Build history of the part. All positions in model axes, mm. A direction names the side the tool comes from. Coordinates: 2 decimals unless noted, no trailing zeros. Order: outer loops, then holes, each group sorted by start corner. A loop starts at its lowest first (then second) coordinate and runs counter-clockwise, first axis right, second up. Notation, with made-up numbers: (64.25, -22.75) -> (123.25, -22.75) arc R16 cw to (123.25, -10.75) -> close; hole circle Ø2 at (-24.5, 14). An arc over 180 degrees is marked (long way). Write each question's results on one line, items separated by ' | '.
from build123d import *
from build123d.topology import SkipClean

# Parameters (mm, degrees)
SKETCH1_W           = 12
SKETCH1_H           = 9
CUT_EXTRUDE1_START  = 1.272656
CUT_EXTRUDE1_DEPTH  = 0.424218618
CUT_EXTRUDE2_DEPTH  = 5.575781382
SKETCH4_R           = 6.3565957
BOSS_EXTRUDE1_DEPTH = 1.811506156
BOSS_EXTRUDE1_TAPER = 11.136309431
SKETCH5_R           = 6
BOSS_EXTRUDE2_DEPTH = 138.188493844
CHAMFER1_SIZE       = 1.0735
FILLET1_R           = 0.6
FILLET2_R           = 1.2


with BuildPart() as part:
    # Sketch1 → Revolve1 (revolve)
    with BuildSketch(Plane.XY, mode=Mode.PRIVATE) as revolve1_sk:
        with Locations((-6, 4.5)):
            Rectangle(SKETCH1_W, SKETCH1_H)
    revolve(revolve1_sk.sketch.rotate(Axis((-12, 0, 0), (1, 0, 0)), 270), axis=Axis((-12, 0, 0), (1, 0, 0)))

    # Sketch2 → Cut-Extrude1 (cut)
    with BuildSketch(Plane.ZY.offset(10.727344145).offset(CUT_EXTRUDE1_START)):
        Polygon((-2.541695199, 4.306054284), (-2.494007969, 4.33358652), (-2.458304232, 4.354200082), (0, 5.773502692), (2.458305244, 4.354200082), (2.505992237, 4.326667984), (2.541695697, 4.306054284), (5, 2.886751346), (5, 0.048145191), (5, -0.00115583), (5, -0.048145419), (5, -2.886751346), (2.541695697, -4.306053956), (2.494008981, -4.333586191), (2.458305244, -4.354199753), (0, -5.773502692), (-2.458304232, -4.354199753), (-2.505991462, -4.326667518), (-2.541695199, -4.306053956), (-5, -2.886751346), (-5, -0.048145419), (-5, -0.00115583), (-5, 0.048145191), (-5, 2.886751346), align=None)
    extrude(amount=-CUT_EXTRUDE1_DEPTH, mode=Mode.SUBTRACT)

    # Sketch3 → Cut-Extrude2 (cut)
    with SkipClean():  # the faces are left unmerged after this step: merging them gives an invalid solid
        with BuildSketch(Plane.ZY.offset(11.575781382)):
            Polygon((0, 5.773502692), (-5, 2.886751346), (-5, -2.886751346), (0, -5.773502692), (5, -2.886751346), (5, 2.886751346), align=None)
        extrude(amount=-CUT_EXTRUDE2_DEPTH, mode=Mode.SUBTRACT)

    # Sketch4 → Boss-Extrude1 (add)
    with SkipClean():  # the faces are left unmerged after this step: merging them gives an invalid solid
        with BuildSketch(Plane(origin=(0, 0, 0), x_dir=(0, 0, -1), z_dir=(1, 0, 0))):
            Circle(SKETCH4_R)
        extrude(amount=BOSS_EXTRUDE1_DEPTH, taper=BOSS_EXTRUDE1_TAPER)

    # Sketch5 → Boss-Extrude2 (add)
    with SkipClean():  # the faces are left unmerged after this step: merging them gives an invalid solid
        with BuildSketch(Plane(origin=(1.811506156, 0, 0), x_dir=(0, 0, -1), z_dir=(1, 0, 0))):
            Circle(SKETCH5_R)
        extrude(amount=BOSS_EXTRUDE2_DEPTH)

    # Sketch6 → Cut-Revolve1 (revolve, cut)
    with SkipClean():  # the faces are left unmerged after this step: merging them gives an invalid solid
        with BuildSketch(Plane.XY, mode=Mode.PRIVATE) as cut_revolve1_sk:
            Polygon((-6, 5), (-6, 0), (-3.113248654, 0), align=None)
        revolve(cut_revolve1_sk.sketch.rotate(Axis((-6, 0, 0), (1, 0, 0)), 90), axis=Axis((-6, 0, 0), (1, 0, 0)), mode=Mode.SUBTRACT)

    # Chamfer1
    chamfer1_edges = [part.edges().sort_by_distance(p)[0] for p in [
        (140, 0, 6),
    ]]
    chamfer(chamfer1_edges, length=CHAMFER1_SIZE)

    # Fillet1
    fillet1_edges = [part.edges().sort_by_distance(p)[0] for p in [
        (0, 0, 6.3565957),
        (1.811506156, 0, 6),
    ]]
    fillet(fillet1_edges, radius=FILLET1_R)

    # Fillet2
    fillet2_edges = [part.edges().sort_by_distance(p)[0] for p in [
        (-12, 0, 9),
    ]]
    fillet(fillet2_edges, radius=FILLET2_R)


solid = part.part
Item 1: Pull direction Y, two halves, no side cores. Call faces 4 (the flat face through (-6, 2.7, 4.5)), 5 (the cylindrical face through (-5.324, 2.703, -8.584)), 6 (the flat face through (0, -7, -2)): released by +Y, released by -Y, zero draft, split by the parting line, or undercut.
Answer:
face 4: undercut | face 5: split by the parting line | face 6: zero draft
Item 2: Drill centre lines: line 1 (X direction, y = -5.75, z = 5); line 2 (Y direction, x = 87, z = -0.5); line 3 (Z direction, x = 134, y = 0.25). Where is each one in solid material? Low to high. Write a range as from..to.
Answer:
line 1: x = -12..0 | line 2: y = -5.98..5.98 | line 3: z = -5.99..5.99
Item 3: Tool access for faces 1 (the flat face through (-6, -2.6, 4.5)), 2 (the flat face through (140, 0, 0)), 3 (the cylindrical face through (69, 0, 6)): list every direction of +Z, -Z, +X, -X, +Y, -Y with a clear straight run to the whole face (end or side of a thin tool).
Answer:
face 1: -X | face 2: +Z, -Z, +X, +Y, -Y | face 3: +X
Item 4: Slice it at A-A, the plane x = 62. List the corners of the cut face in (y, z), and give its area (3 significant figures).
Answer:
outline: circle Ø12 at (0, 0) | area: 113 mm^2
Item 5: Pin check, flat tips, straight feed: pin 1 (0.8 mm diameter, centred on y = -1.5, z = -3.5, fed in from -X); pin 2 (0.7 mm diameter, centred on y = 5, z = -0.5, fed in from -X); pin 3 (4 mm diameter, centred on x = 120, z = 2.5, fed in from -Y). Stop position of each tip, or through.
Answer:
pin 1: stops at x = -5.54 | pin 2: stops at x = -6 | pin 3: stops at y = -5.98
